```python
from build123d import *

# Parameters (mm, degrees)
SKETCH3_W           = 13.4
SKETCH3_H           = 13.4
BOSS_EXTRUDE2_DEPTH = 0.5
SKETCH4_W           = 12
SKETCH4_H           = 12
BOSS_EXTRUDE3_DEPTH = 4


with BuildPart() as part:
    # Sketch3 → Boss-Extrude2 (new body)
    with BuildSketch(Plane(origin=(0, 0, 0), x_dir=(1, 0, 0), z_dir=(0, 1, 0))):
        Rectangle(SKETCH3_W, SKETCH3_H)
    extrude(amount=BOSS_EXTRUDE2_DEPTH)

    # Sketch4 → Boss-Extrude3 (add)
    with BuildSketch(Plane(origin=(0, 0, 0), x_dir=(1, 0, 0), z_dir=(0, 1, 0))):
        Rectangle(SKETCH4_W, SKETCH4_H)
    extrude(amount=BOSS_EXTRUDE3_DEPTH)


solid = part.part
```
Check sheet for the modelled part. Datum: model origin and axes. Units: mm. A direction names the side the tool comes from. Round coordinates to 2 decimals unless told otherwise and drop trailing zeros. Loops run counter-clockwise (first coordinate to the right, second up) from the corner with the lowest first, then second, coordinate; pieces in that order, holes last. Notation, with made-up numbers: (65.25, 35.25) - (106.25, 35.25) arc R37 ccw to (106.25, 72.25) - close; hole circle Ø6 at (41, 31). An arc over 180 degrees is marked (long way). Write item = value, one per line. Start each with the question number.
Q1. Depth check by flat-ended pin: P1, Ø1.5, axis at x = -4, y = 3, coming from the +Z side; P2, Ø1.5, axis at y = 3.5, z = -4.5, coming from the +X side; P3, Ø1.8, axis at x = 2.5, y = 2, coming from the -Z side. Enter the tip coordinate at first touch or a pass-through.
Q2. Thickness scan on L1, parallel to X at y = 3.55, z = -4; L2, parallel to Y at x = 6.25, z = 0.5. Record the ranges inside material, lowest first.
Q3. Access from +Z, -Z, +X, -X, +Y, -Y to the whole of each face (thin tool, end or side, straight path). Record for faces 1 (the face through (0, 2, -6)), 2 (the face through (-6, 2, 0)), 3 (the face through (6, 2, 0)), 4 (the face through (0, 2, 6)).
Q4. Section check B-B (x = 5.5). Record the boundary of the cut face in (y, z), plus the area to 3 significant figures.
Q5. Section check C-C (y = 3.45). Record the boundary of the cut face in (x, z).
Q6. Section check A-A (z = -5.5). Record the boundary of the cut face in (x, y), plus the area to 3 significant figures.
Derived:
q1.P1 = 6
q1.P2 = 6
q1.P3 = -6
q2.L1 = -6 to 6
q2.L2 = 0 to 0.5
q3.face_1 = -Z, +X, -X, +Y
q3.face_2 = +Z, -Z, -X, +Y
q3.face_3 = +Z, -Z, +X, +Y
q3.face_4 = +Z, +X, -X, +Y
q4.outline = (0, -6.7) - (0.5, -6.7) - (0.5, -6) - (4, -6) - (4, 6) - (0.5, 6) - (0.5, 6.7) - (0, 6.7) - close
q4.area = 48.7 mm^2
q5.outline = (-6, -6) - (6, -6) - (6, 6) - (-6, 6) - close
q6.outline = (-6.7, 0) - (6.7, 0) - (6.7, 0.5) - (6, 0.5) - (6, 4) - (-6, 4) - (-6, 0.5) - (-6.7, 0.5) - close
q6.area = 48.7 mm^2
